CAD build for the part. Positions are in the model's coordinates, mm. Give positions to 0.01 mm unless a question says otherwise; leave off trailing zeros. Write each loop counter-clockwise with the first axis right and the second up, starting at its lowest first coordinate (ties: lowest second). Pieces come first, ordered by that corner, then holes. Notation, with made-up numbers: M -3,32.25 L 20,32.25 A19 cw 20,63.25 Z; hole C -4,-40 d5. An arc over 180 degrees is marked long. One line per question, with ' | ' between items. Start each with the question number.
1. Cut at B-B, the plane x = -21. Write the cut outline in (y, z), then the cut area to 3 significant figures.
2. Wall check: L1, parallel to X at y = 2.25, z = 0; L2, parallel to Z at x = 21, y = 0; L3, parallel to Z at x = 25, y = 0.5. Give the ranges that are in metal, low to high.
3. Flat gauge pins, fed straight in: pin 1 (1 mm diameter, centred on x = 6.5, y = -1, fed in from -Z); pin 2 (3 mm diameter, centred on x = -21, z = 0, fed in from -Y); pin 3 (5.5 mm diameter, centred on x = -13.5, z = 1, fed in from +Y); pin 4 (4 mm diameter, centred on x = 5, y = -3.5, fed in from -Z). Where does each tip first touch, or does it go through?
4. Cut at C-C, the plane x = 47. Write the cut outline in (y, z), then the cut area to 3 significant figures.
5. Cut at A-A, the plane y = 0.5. Write the cut outline in (x, z), then the cut area to 3 significant figures.
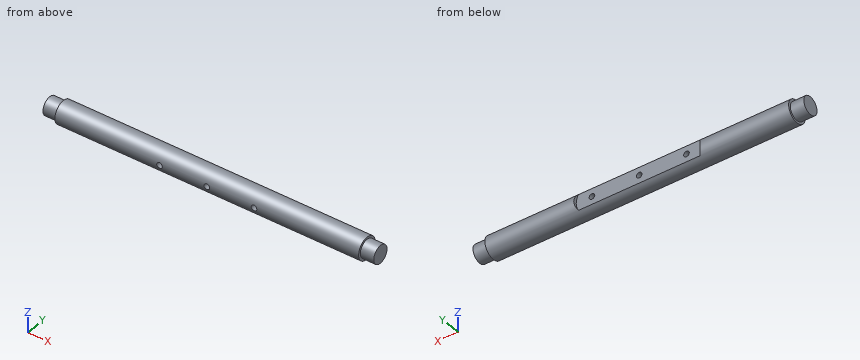
```python
from build123d import *

# Parameters (mm, degrees)
ENL_V_MAT_EXTRU_1_DEPTH      = 74.839352652
ENL_V_MAT_EXTRU_1_DEPTH_BACK = 74.839352652
ESQUISSE2_R                  = 1.25
ENL_V_START                  = 3.5
ENL_V_MAT_EXTRU_2_DEPTH      = 10


with BuildPart() as part:
    # Esquisse1 → Révolution1 (revolve)
    with BuildSketch(Plane.XY):
        Polygon((-67.5, 5), (67.5, 5), (67.5, 4), (73.5, 4), (73.5, 0), (-73.5, 0), (-73.5, 4), (-67.5, 4), align=None)
    revolve(axis=Axis((-73.5, 0, 0), (-1, 0, 0)))

    # Esquisse2 → Enlèv. mat.-Extru.1 (cut, two sides: drawn at the far end of the back side and taken through both)
    with BuildSketch(Plane(origin=(0, 0, 0), x_dir=(1, 0, 0), z_dir=(0, 1, 0)).offset(-ENL_V_MAT_EXTRU_1_DEPTH_BACK)):
        with Locations(Location((-21, 0, 0), (0, 0, 270))):
            Circle(ESQUISSE2_R)
        with Locations(Location((21, 0, 0), (0, 0, 270))):
            Circle(ESQUISSE2_R)
        with Locations(Location((0, 0, 0), (0, 0, 270))):
            Circle(ESQUISSE2_R)
    extrude(amount=ENL_V_MAT_EXTRU_1_DEPTH + ENL_V_MAT_EXTRU_1_DEPTH_BACK, mode=Mode.SUBTRACT)

    # Esquisse3 → Enlèv. mat.-Extru.2 (cut)
    with BuildSketch(Plane(origin=(0, 0, 0), x_dir=(1, 0, 0), z_dir=(0, 1, 0)).offset(ENL_V_START)):
        with BuildLine():
            Line((-21, 7), (21, 7))
            ThreePointArc((21, 7), (28, 0), (21, -7))
            Line((21, -7), (-21, -7))
            ThreePointArc((-21, -7), (-28, 0), (-21, 7))
        make_face()
    extrude(amount=ENL_V_MAT_EXTRU_2_DEPTH, mode=Mode.SUBTRACT)


solid = part.part
```
Here are the results:
1) outline: M -4.84,-1.25 A5 ccw 3.5,-3.57 L 3.5,-1.25 Z; M -4.84,1.25 L 3.5,1.25 L 3.5,3.57 A5 ccw Z | area: 50.0 mm^2
2) L1: -73.5 to -22.25, -19.75 to -1.25, 1.25 to 19.75, 22.25 to 73.5 | L2: -5 to -1.25, 1.25 to 5 | L3: -4.97 to 4.97
3) pin 1: z = -4.97 | pin 2: y = -5 | pin 3: y = 3.5 | pin 4: z = -4.77
4) outline: C 0,0 d10 | area: 78.5 mm^2
5) outline: M -73.5,-3.97 L -67.5,-3.97 L -67.5,-4.97 L 67.5,-4.97 L 67.5,-3.97 L 73.5,-3.97 L 73.5,3.97 L 67.5,3.97 L 67.5,4.97 L -67.5,4.97 L -67.5,3.97 L -73.5,3.97 Z; hole C -21,0 d2.5; hole C 0,0 d2.5; hole C 21,0 d2.5 | area: 1,420 mm^2
